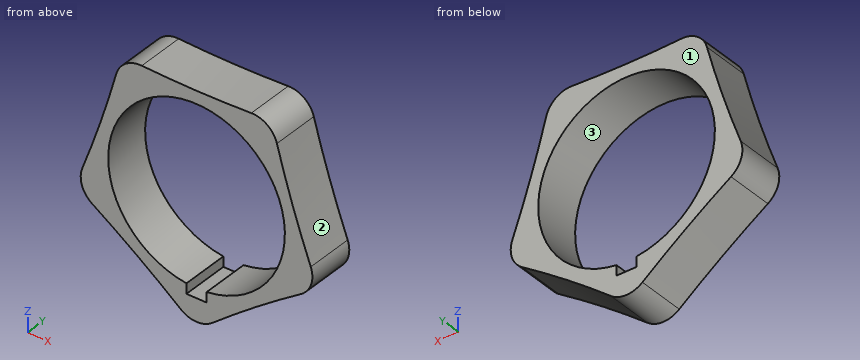
from build123d import *

# Parameters (mm, degrees)
F0_R     = 17.5
F1_DEPTH = 9.5
F2_R     = 5
F4_DEPTH = 9.5010001


with BuildPart() as f1:
    # F0 (on Front) → F1 (new body)
    with BuildSketch(Plane.XZ):
        with BuildLine():
            ThreePointArc((24.099195344, -7.8303032306), (19.0211303259, 6.1803398875), (14.8941218241, 20.5))
            ThreePointArc((14.8941218241, 20.5), (0, 20), (-14.8941218241, 20.5))
            ThreePointArc((-14.8941218241, 20.5), (-19.0211303259, 6.1803398875), (-24.099195344, -7.8303032306))
            ThreePointArc((-24.099195344, -7.8303032306), (-11.7557050458, -16.1803398875), (0, -25.3393935387))
            ThreePointArc((0, -25.3393935387), (11.7557050458, -16.1803398875), (24.099195344, -7.8303032306))
        make_face()
        Circle(F0_R, mode=Mode.SUBTRACT)
    extrude(amount=F1_DEPTH)

    # F2
    f2_edges = [f1.edges().sort_by_distance(p)[0] for p in [
        (0, -4.75, -25.339394),
        (-24.099195, -4.75, -7.830303),
        (-14.894122, -4.75, 20.5),
        (14.894122, -4.75, 20.5),
        (24.099195, -4.75, -7.830303),
    ]]
    fillet(f2_edges, radius=F2_R)

    # F3 (on face) → F4 (cut, through all)
    with BuildSketch(Plane.XZ.offset(9.5)):
        Polygon((2, -19.3853386507), (2, -17.3853386507), (-2, -17.3853386507), (-2, -19.3853386507), (0, -19.3853386507), align=None)
    extrude(amount=-F4_DEPTH, mode=Mode.SUBTRACT)


solid = f1.part
Geometry check sheet. Reference: the model listing, model coordinates, mm. Face numbers are marked on the shaded views. Coordinates: 2 decimals unless noted, no trailing zeros. Loops run counter-clockwise (first coordinate to the right, second up) from the corner with the lowest first, then second, coordinate; pieces in that order, holes last. Notation, with made-up numbers: (55, 43) - (91, 43) arc R12 ccw to (91, 55) - close; hole circle Ø2 at (59, -26.5). An arc over 180 degrees is marked (long way). Use one line per item in the form item = value. Start each with the question number.
Item 1: Section check C-C, the plane x = 19. Enter the section's corners in (y, z).
Item 2: Thickness scan on probe 1 along Z at (x, y) = (0, -6.25); probe 2 along Z at (x, y) = (-9, -1); probe 3 along X at (y, z) = (-8.75, -3). Record the ranges inside material, lowest first.
Item 3: Mould release check, pull along Z, two halves, no side actions. Record for the marked faces 1, 2 and 3: +Z half, -Z half, draft (parallel to the pull), parting line (faces both ways), or undercut.
Item 4: Section check A-A, the plane z = -2. Enter the section's corners in (x, y).
Item 5: Gauge pin test, flat ends, axial feed: pin 1 (2 mm diameter, centred on y = -7, z = -18, fed in from +X); pin 2 (0.6 mm diameter, centred on y = -3.5, z = -18.5, fed in from -X); pin 3 (1.5 mm diameter, centred on x = 3.5, y = -2.5, fed in from +Z). Record the tip position at first contact, or that the pin passes through.
Item 6: Section check B-B, the plane x = -16.5. Enter the section's corners in (y, z).
Computed:
q1.outline = (-9.5, -11.13) - (0, -11.13) - (0, 6.25) - (-9.5, 6.25) - close
q2.probe_1 = -23.88 to -19.39, 17.5 to 20
q2.probe_2 = -18.22 to -15.01, 15.01 to 20.18
q2.probe_3 = -22.23 to -17.24, 17.24 to 22.23
q3.face_1 = draft
q3.face_2 = +Z half
q3.face_3 = undercut
q4.outline = (-21.86, -9.5) - (-17.39, -9.5) - (-17.39, 0) - (-21.86, 0) - close; (17.39, -9.5) - (21.86, -9.5) - (21.86, 0) - (17.39, 0) - close
q5.pin_1 = 10.63
q5.pin_2 = -9.02
q5.pin_3 = 20.04
q6.outline = (-9.5, -12.83) - (0, -12.83) - (0, -5.83) - (-9.5, -5.83) - close; (-9.5, 5.83) - (0, 5.83) - (0, 14.49) - (-9.5, 14.49) - close
